from build123d import *

# Parameters (mm, degrees)
SKETCH1_W                       = 50
SKETCH1_H                       = 50
BOSS_EXTRUDE1_DEPTH             = 50
SKETCH3_W                       = 45
SKETCH3_H                       = 45
CUT_EXTRUDE4_DEPTH              = 45
SKETCH5_R                       = 3
BOSS_EXTRUDE2_DEPTH             = 8
TAP_DRILL_FOR_M3X0_5_TAP2_D     = 2.5
TAP_DRILL_FOR_M3X0_5_TAP2_DEPTH = 8
TAP_DRILL_FOR_M3X0_5_TAP2_TIP   = 0.751075774
SKETCH10_R                      = 6
CUT_EXTRUDE5_DEPTH              = 5
FILLET2_R                       = 5


with BuildPart() as part:
    # Sketch1 → Boss-Extrude1 (new body)
    with BuildSketch(Plane.XY):
        Rectangle(SKETCH1_W, SKETCH1_H)
    extrude(amount=-BOSS_EXTRUDE1_DEPTH)

    # Sketch3 → Cut-Extrude4 (cut)
    with BuildSketch(Plane.XY):
        Rectangle(SKETCH3_W, SKETCH3_H)
    extrude(amount=-CUT_EXTRUDE4_DEPTH, mode=Mode.SUBTRACT)

    # Sketch5 → Boss-Extrude2 (add)
    with BuildSketch(Plane.XY.offset(-45)):
        with Locations((-14.5, 0)):
            Circle(SKETCH5_R)
        with Locations((14.5, 0)):
            Circle(SKETCH5_R)
    extrude(amount=BOSS_EXTRUDE2_DEPTH)

    # Tap Drill for M3x0.5 Tap2
    with Locations(Plane.XY.offset(-37)):
        with Locations((-14.5, 0), (14.5, 0)):
            Hole(TAP_DRILL_FOR_M3X0_5_TAP2_D / 2, depth=TAP_DRILL_FOR_M3X0_5_TAP2_DEPTH)
            with Locations((0, 0, -(TAP_DRILL_FOR_M3X0_5_TAP2_DEPTH + TAP_DRILL_FOR_M3X0_5_TAP2_TIP / 2))):  # 118° drill point
                Cone(0, TAP_DRILL_FOR_M3X0_5_TAP2_D / 2, TAP_DRILL_FOR_M3X0_5_TAP2_TIP, mode=Mode.SUBTRACT)

    # Sketch10 → Cut-Extrude5 (cut)
    with BuildSketch(Plane(origin=(0, -22.5, 0), x_dir=(1, 0, 0), z_dir=(0, 1, 0))):
        with Locations((0, 38.184638056)):
            Circle(SKETCH10_R)
    extrude(amount=-CUT_EXTRUDE5_DEPTH, mode=Mode.SUBTRACT)

    # Fillet2
    fillet2_edges = [part.edges().sort_by_distance(p)[0] for p in [
        (22.5, 22.5, -22.5),
        (22.5, -22.5, -22.5),
        (-22.5, -22.5, -22.5),
        (-22.5, 22.5, -22.5),
        (25, -25, -25),
        (-25, -25, -25),
        (-25, 25, -25),
        (25, 25, -25),
    ]]
    fillet(fillet2_edges, radius=FILLET2_R)


solid = part.part
Design review of the part built by this model. Coordinates are the model's own, in mm. A direction names the side the tool comes from. Round coordinates to 2 decimals unless told otherwise and drop trailing zeros. Loops run counter-clockwise (first coordinate to the right, second up) from the corner with the lowest first, then second, coordinate; pieces in that order, holes last. Notation, with made-up numbers: M 30.5,85.25 L 37.5,85.25 A17 cw 37.5,91.25 Z; hole C -23.5,48 d10. An arc over 180 degrees is marked long. Answer as a JSON object with one key per item and string values.
Item 1: We need section D-D on y = 21. Give the boundary of the cut face in (x, z).
Answer sheet:
{"outline": "M -24.9,-50 L 24.9,-50 L 24.9,0 L 21.07,0 L 21.07,-45 L -21.07,-45 L -21.07,0 L -24.9,0 Z"}
Item 2: We need section C-C on z = -42. Give the boundary of the cut face in (x, y).
Answer sheet:
{"outline": "M -25,-20 A5 ccw -20,-25 L -4.63,-25 L -4.63,-22.5 L -17.5,-22.5 A5 cw -22.5,-17.5 L -22.5,17.5 A5 cw -17.5,22.5 L 17.5,22.5 A5 cw 22.5,17.5 L 22.5,-17.5 A5 cw 17.5,-22.5 L 4.63,-22.5 L 4.63,-25 L 20,-25 A5 ccw 25,-20 L 25,20 A5 ccw 20,25 L -20,25 A5 ccw -25,20 Z; C -14.5,0 d6; C 14.5,0 d6; hole C -14.5,0 d2.5; hole C 14.5,0 d2.5"}
Item 3: Clearance check with flat-ended pins moving along their axes: P1, Ø13.5, axis at x = 4, y = 5, coming from the +Z side; P2, Ø1.8, axis at x = -15.5, y = 1, coming from the +Z side. State where each tip first meets the part, or that it passes through.
Answer sheet:
{"P1": "stops at z = -45", "P2": "stops at z = -37"}
Item 4: The part is to be moulded in two halves that separate along X. For faces 1 (the flat face through (0, -25, -25)), 2 (the cylindrical face through (-24, 23, -25)), 3 (the flat face through (25, 0, -25)), 4 (the cylindrical face through (21, -21.07, -22.82)), say which applies: pulls with the +X half, pulls with the -X half, needs draft (parallel to the pull), parting line crosses it, or undercut.
Answer sheet:
{"face 1": "needs draft", "face 2": "pulls with the -X half", "face 3": "pulls with the +X half", "face 4": "undercut"}
Item 5: Wall thickness on L1, parallel to Y at x = 14.5, z = -41; L2, parallel to Y at x = -16, z = -19.5; L3, parallel to Z at x = 0, y = -23.15: over which ranges is each line inside the solid? List them lowest first. Write a range as from..to.
Answer sheet:
{"L1": "y = -25..-22.5, -3..-1.25, 1.25..3, 22.5..25", "L2": "y = -25..-22.5, 22.5..25", "L3": "z = -50..-44.18, -32.18..0"}
Item 6: Machinability: for faces 5 (the flat face through (0, 0, -50)), 6 (the flat face through (0, -22.5, -22)), which of the approach directions +Z, -Z, +X, -X, +Y, -Y give a long, thin tool a straight path to every point of the face, cutting with its end or side? Answer none if there is none.
Answer sheet:
{"face 5": "-Z, +X, -X, +Y, -Y", "face 6": "+Z"}
Item 7: We need section B-B on x = 0. Give the boundary of the cut face in (y, z).
Answer sheet:
{"outline": "M -25,-50 L 25,-50 L 25,0 L 22.5,0 L 22.5,-45 L -22.5,-45 L -22.5,-44.18 L -25,-44.18 Z; M -25,-32.18 L -22.5,-32.18 L -22.5,0 L -25,0 Z"}
Item 8: We need section A-A on z = -27. Give the boundary of the cut face in (x, y), and give its area (3 significant figures).
Answer sheet:
{"outline": "M -25,-20 A5 ccw -20,-25 L 20,-25 A5 ccw 25,-20 L 25,20 A5 ccw 20,25 L -20,25 A5 ccw -25,20 Z; hole M -22.5,-17.5 A5 ccw -17.5,-22.5 L 17.5,-22.5 A5 ccw 22.5,-17.5 L 22.5,17.5 A5 ccw 17.5,22.5 L -17.5,22.5 A5 ccw -22.5,17.5 Z", "area": "475 mm^2"}
